from build123d import *

# Parameters (mm, degrees)
DOME1_FACE_RADIUS  = 20
DOME1_HEIGHT       = 20
SKETCH3_OUTSIDE_W  = 177.57
SKETCH3_OUTSIDE_H  = 177.57
CUT_EXTRUDE4_DEPTH = 236.796522451
SKETCH5_OUTSIDE_W  = 447.476
SKETCH5_OUTSIDE_H  = 431.4
SKETCH5_OUTSIDE_R  = 51.961524227
CUT_EXTRUDE5_DEPTH = 234.880311271
CUT_EXTRUDE5_DRAFT = -30


with BuildPart() as part:
    # Sketch1 → Revolve2 (revolve)
    with BuildSketch(Plane(origin=(0, 0, 0), x_dir=(1, 0, 0), z_dir=(0, 1, 0)), mode=Mode.PRIVATE) as revolve2_sk:
        Polygon((0, 0), (0, 60), (60, 60), (60, 30), (160, 30), (160, 20), (200, 20), (200, 0), align=None)
    revolve(revolve2_sk.sketch.rotate(Axis((0, 0, 0), (1, 0, 0)), 180), axis=Axis((0, 0, 0), (1, 0, 0)))

    # Dome1: a dome of height H over a round flat face of radius A is a cap of a sphere of radius (A * A + H * H) / (2 * H)
    dome1_r = (DOME1_FACE_RADIUS * DOME1_FACE_RADIUS + DOME1_HEIGHT * DOME1_HEIGHT) / (2 * DOME1_HEIGHT)
    dome1_base = Plane((200, 0, 0), z_dir=(1, 0, 0))
    with Locations(dome1_base.offset(DOME1_HEIGHT - dome1_r)):
        dome1_ball = Sphere(dome1_r, mode=Mode.PRIVATE)
    add(split(dome1_ball, bisect_by=dome1_base, keep=Keep.TOP, mode=Mode.PRIVATE))

    # Sketch3 outside → Cut-Extrude4 (cut, through all)
    with BuildSketch(Plane.ZY):
        Rectangle(SKETCH3_OUTSIDE_W, SKETCH3_OUTSIDE_H)
        Polygon((60, 0), (30, 51.961524227), (-30, 51.961524227), (-60, 0), (-30, -51.961524227), (30, -51.961524227), align=None, mode=Mode.SUBTRACT)
    extrude(amount=-CUT_EXTRUDE4_DEPTH, mode=Mode.SUBTRACT)


with BuildPart() as cut_extrude5_tool:
    # Sketch5 outside → Cut-Extrude5 (with draft: the straight prism first)
    with BuildSketch(Plane.ZY):
        Rectangle(SKETCH5_OUTSIDE_W, SKETCH5_OUTSIDE_H)
        Circle(SKETCH5_OUTSIDE_R, mode=Mode.SUBTRACT)
    extrude(amount=-CUT_EXTRUDE5_DEPTH)
    # Cut-Extrude5: the draft: its side faces are tilted about the plane it starts from
    cut_extrude5_sides = [cut_extrude5_tool.faces().sort_by_distance(p)[0] for p in [
        (117.440155635, -215.7, 0),
        (117.440155635, 0, 223.738),
        (117.440155635, 215.7, 0),
        (117.440155635, 0, -223.738),
        (117.440155635, 0, -51.961524227),
    ]]
    draft(cut_extrude5_sides, Plane.ZY, CUT_EXTRUDE5_DRAFT)


with BuildPart() as part_1:
    add(part.part)

    # Cut-Extrude5: cut by cut_extrude5_tool
    add(cut_extrude5_tool.part, mode=Mode.SUBTRACT)


solid = part_1.part
Geometry: final body of the model. Coordinates: model frame, mm. A direction names the side the tool comes from. Coordinates: 2 decimals unless noted, no trailing zeros. Order: outer loops, then holes, each group sorted by start corner. A loop starts at its lowest first (then second) coordinate and runs counter-clockwise, first axis right, second up. Notation, with made-up numbers: (2, 44.25) - (13, 44.25) arc R26 cw to (13, 59.25) - close; hole circle Ø3 at (59.5, 11.5). An arc over 180 degrees is marked (long way). Use one line per item in the form item = value.
1) Ray query, L1, parallel to X at y = 18, z = -20; L2, parallel to X at y = -28, z = 35; L3, parallel to Y at x = 24.5, z = 53.5. Return the intervals inside material, ascending.
Solutions:
L1 = 0 to 160
L2 = 0 to 60
L3 = -11.26 to 11.26
2) Section B-B (x = 176). Return loops of the section in (y, z).
Solutions:
outline = circle Ø40 at (0, 0)
3) Section C-C (x = 151). Return loops of the section in (y, z).
Solutions:
outline = circle Ø60 at (0, 0)
4) Set-up query: faces 1 (the face through (180.28, -0.88, -19.98)), 2 (the face through (30, -51.962, 0)). Return all of +Z, -Z, +X, -X, +Y, -Y with unobstructed straight access to the full face (end or side cutting, diameter ignored); none if empty.
Solutions:
face_1 = +X
face_2 = +Z, -Z, +X, -X, -Y
5) Pin query (flat end, axial travel): pin 1 (10 mm diameter, centred on y = -28.5, z = -29, fed in from -X); pin 2 (1.5 mm diameter, centred on y = 9, z = 24.5, fed in from +X); pin 3 (6 mm diameter, centred on x = 154, z = 33.5, fed in from +Y); pin 4 (2 mm diameter, centred on x = 49, z = 37, fed in from +Y). Return the tip coordinate at first contact, or that it passes through.
Solutions:
pin_1 = 0
pin_2 = 160
pin_3 = through
pin_4 = 41.57
6) Section A-A (x = 41). Return loops of the section in (y, z), then the cut area to 3 significant figures.
Solutions:
outline = (-51.96, -30) - (0, -60) - (51.96, -30) - (51.96, 30) - (0, 60) - (-51.96, 30) - close
area = 9,350 mm^2
